```python
from build123d import *

# Parameters (mm, degrees)
SKETCH1_R           = 4
SKETCH1_R_2         = 1.5
BOSS_EXTRUDE1_DEPTH = 2
SKETCH2_R           = 4
SKETCH2_R_2         = 1.5
BOSS_EXTRUDE2_DEPTH = 2
FILLET1_R           = 2


with BuildPart() as part:
    # Sketch1 → Boss-Extrude1 (new body)
    with BuildSketch(Plane.XY):
        with BuildLine():
            Line((-12.5, 0), (-12.5, -19.5))
            Line((-12.5, -19.5), (12.5, -19.5))
            Line((12.5, -19.5), (12.5, 0))
            ThreePointArc((12.5, 0), (0, 12.5), (-12.5, 0))
        make_face()
        Circle(SKETCH1_R, mode=Mode.SUBTRACT)
        with Locations((0, 7)):
            Circle(SKETCH1_R_2, mode=Mode.SUBTRACT)
        with Locations((7, 0)):
            Circle(SKETCH1_R_2, mode=Mode.SUBTRACT)
        with Locations((0, -7)):
            Circle(SKETCH1_R_2, mode=Mode.SUBTRACT)
        with Locations((-7, 0)):
            Circle(SKETCH1_R_2, mode=Mode.SUBTRACT)
    extrude(amount=-BOSS_EXTRUDE1_DEPTH)

    # Sketch2 → Boss-Extrude2 (add)
    with BuildSketch(Plane.XZ.offset(19.5)):
        with BuildLine():
            Line((-12.5, -16), (-12.5, 0))
            Line((-12.5, 0), (12.5, 0))
            Line((12.5, 0), (12.5, -16))
            ThreePointArc((12.5, -16), (0, -28.5), (-12.5, -16))
        make_face()
        with Locations((0, -16)):
            Circle(SKETCH2_R, mode=Mode.SUBTRACT)
        with Locations((0, -9)):
            Circle(SKETCH2_R_2, mode=Mode.SUBTRACT)
        with Locations((7, -16)):
            Circle(SKETCH2_R_2, mode=Mode.SUBTRACT)
        with Locations((0, -23)):
            Circle(SKETCH2_R_2, mode=Mode.SUBTRACT)
        with Locations((-7, -16)):
            Circle(SKETCH2_R_2, mode=Mode.SUBTRACT)
    extrude(amount=-BOSS_EXTRUDE2_DEPTH)

    # Fillet1
    fillet1_edges = [part.edges().sort_by_distance(p)[0] for p in [
        (0, -17.5, -2),
        (0, -19.5, 0),
    ]]
    fillet(fillet1_edges, radius=FILLET1_R)


solid = part.part
```
Here's how the part is built. I have some questions about the finished solid (model axes, mm). A direction names the side the tool comes from. Coordinates: 2 decimals unless noted, no trailing zeros. Write each loop counter-clockwise with the first axis right and the second up, starting at its lowest first coordinate (ties: lowest second). Pieces come first, ordered by that corner, then holes. Notation, with made-up numbers: (-26.75, 34.25) -> (-7.75, 34.25) arc R28 ccw to (-7.75, 55.25) -> close; hole circle Ø7 at (26.5, -24.5). An arc over 180 degrees is marked (long way). Use a Markdown table: item, result. Add a question column.
(1) If we section it at C-C, the plane x = 0: State how many separate pieces and enclosed holes the cut face has, and give its area (3 significant figures).
(2) For faces 1 (the cylindrical face through (5.5, 0.07, -0.99)), 2 (the flat face through (-0.2, -4.4, -2)), which set-ups out of +Z, -Z, +X, -X, +Y, -Y let a thin tool reach every point of the face, with its end or its side?
(3) We'd pull the mould along X, two halves only. Please class faces 3 (the cylindrical face through (0.275, -18.514, -28.497)), 4 (the cylindrical face through (-0.867, -3.905, -0.986)), 5 (the cylindrical face through (-8.5, 0.07, -0.99)), 6 (the flat face through (3, -19.5, -12)): +X half, -X half, draft (parallel to the pull), parting line (faces both ways), or undercut.
(4) I'm going to push flat-ended pins straight in: P1, Ø5, axis at x = 7, y = 0, coming from the -Z side; P2, Ø1.5, axis at x = 5, z = -12.5, coming from the +Y side; P3, Ø13, axis at x = 0, y = 0, coming from the +Z side; P4, Ø6, axis at y = 2.5, z = -4, coming from the +X side. Where does each tip first touch, or does it pass through?
(5) If we section it at D-D, the plane x = -6.5: Write out the boundary of the cut face in (y, z), and give its area (3 significant figures).
(6) Please list where these lines run through material, in increasing order: line 1 (Z direction, x = 1, y = -10); line 2 (Y direction, x = -4.75, z = -23); line 3 (X direction, y = 6, z = -1.75).
(7) If we section it at A-A, the plane y = -7: Write out the boundary of the cut face in (x, z), and give its area (3 significant figures).
(8) If we section it at B-B, the plane z = -9: Write out the boundary of the cut face in (x, y), and give its area (3 significant figures).
Outcome:
| question | item | result |
|---|---|---|
| 1 | separate pieces | 7 |
| 1 | enclosed holes | 0 |
| 1 | area | 61.0 mm^2 |
| 2 | face 1 | +Z, -Z |
| 2 | face 2 | -Z, +X, -X, +Y |
| 3 | face 3 | parting line |
| 3 | face 4 | undercut |
| 3 | face 5 | undercut |
| 3 | face 6 | draft |
| 4 | P1 | stops at z = -2 |
| 4 | P2 | stops at y = -17.5 |
| 4 | P3 | stops at z = 0 |
| 4 | P4 | stops at x = 12.5 |
| 5 | outline | (-19.5, -26.68) -> (-17.5, -26.68) -> (-17.5, -17.41) -> (-19.5, -17.41) -> close; (-19.5, -14.59) -> (-17.5, -14.59) -> (-17.5, -4) arc R2 cw to (-15.5, -2) -> (-1.41, -2) -> (-1.41, 0) -> (-17.5, 0) arc R2 ccw to (-19.5, -2) -> close; (1.41, -2) -> (10.68, -2) -> (10.68, 0) -> (1.41, 0) -> close |
| 5 | area | 98.4 mm^2 |
| 6 | line 1 | z = -2 to 0 |
| 6 | line 2 | y = -19.5 to -17.5 |
| 6 | line 3 | x = -10.97 to -1.12, 1.12 to 10.97 |
| 7 | outline | (-12.5, -2) -> (-1.5, -2) -> (-1.5, 0) -> (-12.5, 0) -> close; (1.5, -2) -> (12.5, -2) -> (12.5, 0) -> (1.5, 0) -> close |
| 7 | area | 44.0 mm^2 |
| 8 | outline | (-12.5, -19.5) -> (-1.5, -19.5) -> (-1.5, -17.5) -> (-12.5, -17.5) -> close; (1.5, -19.5) -> (12.5, -19.5) -> (12.5, -17.5) -> (1.5, -17.5) -> close |
| 8 | area | 44.0 mm^2 |
